Could you check a few things on this model? Use its own coordinates, in mm. Round coordinates to 2 decimals unless told otherwise and drop trailing zeros. Loops run counter-clockwise (first coordinate to the right, second up) from the corner with the lowest first, then second, coordinate; pieces in that order, holes last. Notation, with made-up numbers: (2, -13.75) -> (22, -13.75) arc R30 cw to (22, 24.25) -> close; hole circle Ø4 at (48, 85). An arc over 180 degrees is marked (long way). Put each result on its own line as item: value. Start each with the question number.
1. I'm going to push a flat-ended pin straight in: P1, Ø5, axis at x = 22.5, z = -5.5, coming from the -Y side. Where does the tip first touch, or does it pass through?
2. I need wall thicknesses on line 1 (Y direction, x = 26.5, z = -8.5); line 2 (X direction, y = 34, z = -2.5); line 3 (Y direction, x = 29.21, z = -9.5). Which ranges of each line are inside material? Lowest first, please. Write a range as [from, to].
3. If we mould it in two halves opening along X, with no side actions, what happens to faces 1 (the flat face through (19, 27, 0)), 2 (the flat face through (0, 21, -6)), 3 (the cylindrical face through (24.126, 5.481, -6.261))? For each: pulls with the +X half, pulls with the -X half, needs draft (parallel to the pull), parting line crosses it, or undercut.
4. Imagine slicing it at B-B, the plane x = 19.05. Please give me the cut outline in (y, z).
5. Imagine slicing it at D-D, the plane z = -5.5. Please give me the cut outline in (x, y).
6. Imagine slicing it at C-C, the plane y = 36.83. Please give me the cut outline in (x, z).
7. Imagine slicing it at A-A, the plane y = 15.24. Please give me the cut outline in (x, z), and give its area (3 significant figures).
```python
from build123d import *

# Parameters (mm, degrees)
SKETCH1_W                        = 38.1
SKETCH1_H                        = 43.18
BOSS_EXTRUDE1_DEPTH              = 12.7
SKETCH3_R                        = 11
CUT_EXTRUDE1_DEPTH               = 13.7
F_17_64_0_26563_DIAMETER_HOLE1_D = 6.747002


with BuildPart() as part:
    # Sketch1 → Boss-Extrude1 (new body)
    with BuildSketch(Plane.XY):
        with Locations((19.05, 21.59)):
            Rectangle(SKETCH1_W, SKETCH1_H)
    extrude(amount=-BOSS_EXTRUDE1_DEPTH)

    # Sketch3 → Cut-Extrude1 (cut, through all)
    with BuildSketch(Plane.XY):
        with Locations((19.05, 15.24)):
            Circle(SKETCH3_R)
    extrude(amount=-CUT_EXTRUDE1_DEPTH, mode=Mode.SUBTRACT)

    # 17/64 (0.26563) Diameter Hole1 (through all)
    with Locations(Plane(origin=(29.21, 36.83, 0), x_dir=(1, 0, 0), z_dir=(0, 0, 1))):
        with Locations((0, 0), (-20.32, 0)):
            Hole(F_17_64_0_26563_DIAMETER_HOLE1_D / 2)


solid = part.part
```
Entries:
1. P1: y = 0
2. line 1: [0, 7.15], [23.33, 34.82], [38.84, 43.18]
2. line 2: [0, 7.05], [10.73, 27.37], [31.05, 38.1]
2. line 3: [0, 11.02], [19.46, 33.46], [40.2, 43.18]
3. face 1: needs draft
3. face 2: pulls with the -X half
3. face 3: undercut
4. outline: (0, -12.7) -> (4.24, -12.7) -> (4.24, 0) -> (0, 0) -> close; (26.24, -12.7) -> (43.18, -12.7) -> (43.18, 0) -> (26.24, 0) -> close
5. outline: (0, 0) -> (38.1, 0) -> (38.1, 43.18) -> (0, 43.18) -> close; hole circle Ø6.75 at (8.89, 36.83); hole circle Ø22 at (19.05, 15.24); hole circle Ø6.75 at (29.21, 36.83)
6. outline: (0, -12.7) -> (5.52, -12.7) -> (5.52, 0) -> (0, 0) -> close; (12.26, -12.7) -> (25.84, -12.7) -> (25.84, 0) -> (12.26, 0) -> close; (32.58, -12.7) -> (38.1, -12.7) -> (38.1, 0) -> (32.58, 0) -> close
7. outline: (0, -12.7) -> (8.05, -12.7) -> (8.05, 0) -> (0, 0) -> close; (30.05, -12.7) -> (38.1, -12.7) -> (38.1, 0) -> (30.05, 0) -> close
7. area: 204 mm^2
